Work out the finished part from the listing and answer in its coordinate system (mm). A direction names the side the tool comes from. Give positions to 0.01 mm unless a question says otherwise; leave off trailing zeros. Loops run counter-clockwise (first coordinate to the right, second up) from the corner with the lowest first, then second, coordinate; pieces in that order, holes last. Notation, with made-up numbers: (57.25, -24.75) - (81.25, -24.75) arc R24 ccw to (81.25, 1.25) - close; hole circle Ø1 at (-33, -12). An arc over 180 degrees is marked (long way). One line per item, written item: value.
Autodesk Inventor part; units mm, degrees
ref_plane "YZ Plane" through (0, 0, 0) normal (1, 0, 0) x (0, 1, 0)
ref_plane "XZ Plane" through (0, 0, 0) normal (0, 1, 0) x (-1, 0, 0)
ref_plane "XY Plane" through (0, 0, 0) normal (0, 0, 1) x (1, 0, 0)
sketch "Sketch1" plane through (0, 0, 0) normal (0, 1, 0) x (-1, 0, 0)
  line L0 (0, 0) -> (-3, 0)
  line L1 (-3, 0) -> (-3, -39)
  line L2 (-3, -39) -> (0, -39)
  line L3 (0, -39) -> (0, 0)
  circle A0 centre (-1.5, 2) radius 2.5
  circle A1 centre (-1.5, 2) radius 1
  dimension "d0" = 39
  dimension "d1" = 3
  dimension "d2" = 5
  dimension "d3" = 2
extrude "Base" add sketch "Sketch1" along normal blind 4
sketch "Sketch2" plane through (0, 4, 0) normal (0, 1, 0) x (1, 0, 0)
  line L0 (0, 39) -> (0, 0)
  line L1 (3, 0) -> (3, 39)
  circle A0 centre (1.5, -2) radius 1
  arc A1 (0, 0) -> (3, 0) centre (1.5, -2) ccw
  line L2 (3, 0) -> (3, 39)
  line L3 (3, 39) -> (0, 39)
  line L4 (0, 39) -> (0, 0)
  line L5 (0, 5) -> (3, 5)
  dimension "d8" = 5
extrude "Superior" add sketch "Sketch2" along normal blind 3 contours L5 L1 A1 L0
fillet "Biselado" radius 1.5 4 edges at (3, 5.5, -5) (0, 5.5, -5) (3, 2, -39) (0, 2, -39)
equation "\"d0\" = traba_largo"
equation "\"d1\" = traba_ancho"
equation "\"d2\" = traba_diametro"
equation "\"d3\" = traba_diametro_perforacion"
equation "\"d4\" = traba_alto"
equation "\"d8\" = traba_top_largo"
equation "\"d9\" = traba_top_alto"
equation "\"d11\" = 0.5 * traba_ancho"
equation "\"base_alto\" = 3"
equation "\"deslizador_alto\" = 3"
equation "\"deslizador_alto_1\" = 3"
equation "\"deslizador_interruptor_ancho\" = 7"
equation "\"deslizador_interruptor_largo\" = 5"
equation "\"deslizador_largo\" = 144"
equation "\"deslizador_saliente\" = 5"
equation "\"deslizador_soporte_alto\" = 4"
equation "\"deslizador_soporte_ancho\" = 5"
equation "\"deslizador_tope_alto\" = 5"
equation "\"hoja_alto\" = 3"
equation "\"hoja_cola_biselado\" = 1"
equation "\"hoja_filo_biselado\" = 0.5"
equation "\"hoja_stop_biselado\" = 2"
equation "\"hoja_stop_largo\" = 5"
equation "\"hoja_stop_posicion\" = 5"
equation "\"hoja_stop_saliente\" = 5"
equation "\"margen\" = 0.3"
equation "\"muros_grosor\" = 3"
equation "\"rail_alto\" = 1.5"
equation "\"rail_grosor\" = 5"
equation "\"tirador_agarre_largo\" = 3"
equation "\"traba_largo\" = 39"
equation "\"traba_ancho\" = 3"
equation "\"traba_diametro\" = 5"
equation "\"traba_diametro_perforacion\" = 2"
equation "\"traba_alto\" = 4"
equation "\"traba_top_largo\" = 5"
equation "\"traba_top_alto\" = 3"
equation "\"base_separacion_agujeros\" = 4"
equation "\"base_agujeros_separacion\" = 3.5"
equation "\"base_agujeros_diametro\" = 2"
properties part number "Traba"
1. For faces 4 (the cylindrical face through (1.6, 3.5, 4.5)), 5 (the cylindrical face through (0.45, 5.52, -4.57)), 6 (the cylindrical face through (2.57, 5.52, -4.55)), determine the directions among +Z, -Z, +X, -X, +Y, -Y from which every point of the face is accessible in a straight line to the end or side of a thin tool.
Output:
face 4: +Y, -Y
face 5: -Z, -X, +Y
face 6: -Z, +X, +Y
2. Find the intervals of material crossed by line 1 along Z through (x, y) = (1.5, 4.25); line 2 along Z through (x, y) = (1.5, 3); line 3 along X through (y, z) = (2.75, -28.5), in increasing order.
Output:
line 1: z = -5 to 1, 3 to 4.5
line 2: z = -39 to 1, 3 to 4.5
line 3: x = 0 to 3
3. Section B-B (z = 2) is taken. Write down the section's boundary in (x, y), and give its area (3 significant figures).
Output:
outline: (-1, 0) - (0.5, 0) - (0.5, 7) - (-1, 7) - close; (2.5, 0) - (4, 0) - (4, 7) - (2.5, 7) - close
area: 21.0 mm²
4. Section C-C (z = -8) is taken. Write down the section's boundary in (x, y), and give its area (3 significant figures).
Output:
outline: (0, 0) - (3, 0) - (3, 4) - (0, 4) - close
area: 12.0 mm²
5. The mould has two halves that part along X. Classify faces 1 (the flat face through (3, 2, -18)), 2 (the flat face through (0, 2, -19)), 3 (the cylindrical face through (1.434, 3.451, 1.002)): released by +X, released by -X, zero draft, split by the parting line, or undercut.
Output:
face 1: released by +X
face 2: released by -X
face 3: undercut
6. Flat-ended cylindrical pins translate along their axes: pin 1 Ø1.6 at (x, z) = (1.5, 2) entering from -Y; pin 2 Ø2.5 at (x, z) = (2, -18.5) entering from +Y; pin 3 Ø2 at (x, y) = (-0.5, 2) entering from +Z; pin 4 Ø2 at (y, z) = (2, -15) entering from +X. Find the tip coordinate at first contact, or state that the pin passes through.
Output:
pin 1: passes through
pin 2: stops at y = 4
pin 3: stops at z = 4.29
pin 4: stops at x = 3
